Read the model definition and answer for the solid it produces. Units are mm, in the model's axes. A direction names the side the tool comes from. Coordinates: 2 decimals unless noted, no trailing zeros.
1) Find the intervals of material crossed by line 1 (X direction, y = -164.5, z = 1.3); line 2 (Y direction, x = 48, z = 2.05); line 3 (X direction, y = -137.5, z = 0.65), in increasing order.
2) Each of these flat-tipped pins is pushed along its axis until it touches: pin 1 Ø1.5 at (x, z) = (36.5, 1) entering from -Y; pin 2 Ø0.9 at (y, z) = (-146.5, 2) entering from -X; pin 3 Ø0.8 at (x, z) = (0, 1.5) entering from -Y. Where does it stop, or does it pass through?
3) Which of the six approach directions +Z, -Z, +X, -X, +Y, -Y give full straight-line access (tool end or side, diameter ignored) to faces 5 (the face through (-207.952, 49.047, 1.479)), 6 (the face through (146.452, 155.568, 1.479)), 7 (the face through (105, -170, 1))?
4) Determine the mould class of faces 1 (the face through (-148.97, 188.17, 1.48)), 2 (the face through (83.435, 73.401, 1.479)), 3 (the face through (-152, -145, 1)), 4 (the face through (-3, -10, 3)) for opening direction X: +X half, -X half, draft (parallel to the pull), parting line (faces both ways), or undercut.
Autodesk Fusion 360 part; units mm, degrees
sketch "Esboço1" plane through (0, 0, 0) normal (0, 0, 1) x (1, 0, 0)
  circle A0 centre (0, 0) radius 240
  line L0 (48, -48) -> (-48, -48)
  line L1 (-48, -48) -> (-48, 48)
  line L2 (-48, 48) -> (48, 48)
  line L3 (48, 48) -> (48, -48)
  line L4 (48, -48) -> (-48, 48) construction
  line L5 (-48, -48) -> (48, 48) construction
  circle A1 centre (-48, 48) radius 5
  circle A2 centre (-48, -48) radius 5
  circle A3 centre (48, 48) radius 5
  circle A4 centre (48, -48) radius 5
  line L6 (105, -110) -> (105, -170)
  line L7 (90, -125) -> (90, -155)
  line L8 (120, -125) -> (120, -155)
  arc A5 (120, -125) -> (90, -125) centre (105, -125) ccw
  arc A6 (90, -155) -> (120, -155) centre (105, -155) ccw
  circle A7 centre (148, -148) radius 5
  line L9 (-125, 204.878) -> (125, 204.878)
  circle A8 centre (0, 311.043) radius 164
  circle A9 centre (107.5, 130.5) radius 5
  line L10 (-40, 115) -> (40, 115)
  line L11 (-40, 115) -> (-40, 151.9958)
  line L12 (40, 115) -> (40, 151.9958)
  line L13 (0, 1.75) -> (0, 22.5)
  line L14 (-120, -125) -> (-120, -155)
  arc A10 (-90, -125) -> (-120, -125) centre (-105, -125) ccw
  line L15 (-90, -125) -> (-90, -155)
  arc A11 (-120, -155) -> (-90, -155) centre (-105, -155) ccw
  circle A12 centre (-148, -148) radius 5
  circle A13 centre (-107.5, 130.5) radius 5
  line L16 (-61.5, -178) -> (61.5, -178)
  line L17 (61.5, -178) -> (61.5, -240)
  line L18 (61.5, -240) -> (-61.5, -240)
  line L19 (-61.5, -240) -> (-61.5, -178)
  line L20 (0, -178) -> (0, -168)
  line L21 (-37.5, -168) -> (37.5, -168)
  circle A14 centre (-37.5, -168) radius 2.5
  circle A15 centre (37.5, -168) radius 2.5
  circle A16 centre (37.5, -108) radius 2.5
  circle A17 centre (37.5, -48) radius 2.5
  circle A18 centre (-37.5, -108) radius 2.5
  circle A19 centre (-37.5, -48) radius 2.5
  circle A20 centre (126.7423, 116.476) radius 2.5
  line L22 (238.5961, 66.7394) -> (184.9025, 35.7394)
  line L23 (184.9025, 35.7394) -> (123.4025, 142.2606)
  line L24 (123.4025, 142.2606) -> (177.0961, 173.2606)
  circle A21 centre (74.7807, 86.476) radius 2.5
  circle A22 centre (164.2423, 51.524) radius 2.5
  circle A23 centre (112.2807, 21.524) radius 2.5
  circle A24 centre (60.3192, -8.476) radius 2.5
  circle A25 centre (22.8192, 56.476) radius 2.5
  circle A26 centre (-164.2423, 51.524) radius 2.5
  line L25 (-177.0961, 173.2606) -> (-123.4025, 142.2606)
  line L26 (-123.4025, 142.2606) -> (-184.9025, 35.7394)
  line L27 (-184.9025, 35.7394) -> (-238.5961, 66.7394)
  circle A27 centre (-112.2807, 21.524) radius 2.5
  circle A28 centre (-126.7423, 116.476) radius 2.5
  circle A29 centre (-74.7807, 86.476) radius 2.5
  circle A30 centre (-22.8192, 56.476) radius 2.5
  circle A31 centre (-60.3192, -8.476) radius 2.5
  line L28 (0, -178) -> (0, -153)
  line L29 (-22.5, -153) -> (22.5, -153)
  circle A32 centre (-22.5, -153) radius 5
  circle A33 centre (22.5, -153) radius 5
  circle A34 centre (-22.5, -104) radius 5
  circle A35 centre (22.5, -104) radius 5
  circle A36 centre (143.7519, 57.0144) radius 5
  circle A37 centre (101.3166, 32.5144) radius 5
  circle A38 centre (78.8166, 71.4856) radius 5
  circle A39 centre (121.2519, 95.9856) radius 5
  circle A40 centre (-121.2519, 95.9856) radius 5
  circle A41 centre (-78.8166, 71.4856) radius 5
  circle A42 centre (-101.3166, 32.5144) radius 5
  circle A43 centre (-143.7519, 57.0144) radius 5
  line L30 (-17.902, -72) -> (18.098, -72)
  circle A44 centre (-17.902, -72) radius 1.75
  circle A45 centre (18.098, -72) radius 1.75
  line L31 (0, 311.043) -> (0, 115)
  circle A46 centre (-17.902, 74) radius 1.75
  circle A47 centre (18.098, 74) radius 1.75
  point P0 (105, -110)
  point P1 (0, 115)
  point P2 (0, -240)
  point P3 (-61.5, -231.9865)
  point P4 (-170.1562, 169.2538)
  point P5 (170.1562, 169.2538)
  point P6 (0.098, -72)
  dimension "d1" = 480
  dimension "d2" = 96
  dimension "d3" = 96
  dimension "d4" = 10
  dimension "d5" = 10
  dimension "d6" = 10
  dimension "d7" = 10
  dimension "d8" = 110
  dimension "d9" = 105
  dimension "d10" = 30
  dimension "d11" = 60
  dimension "d12" = 30
  dimension "d13" = 10
  dimension "d14" = 148
  dimension "d15" = 148
  dimension "d16" = 250
  dimension "d17" = 328
  dimension "d18" = 10
  dimension "d19" = 130.5
  dimension "d20" = 107.5
  dimension "d21" = 115
  dimension "d22" = 80
  dimension "d25" = 123
  dimension "d26" = 62
  dimension "d27" = 10
  dimension "d28" = 75
  dimension "d29" = 5
  dimension "d30" = 5
  dimension "d33" = 1
  dimension "d34" = 60
  dimension "d36" = 360
  dimension "d37" = 25
  dimension "d38" = 45
  dimension "d39" = 10
  dimension "d40" = 10
  dimension "d43" = 0
  dimension "d44" = 49
  dimension "d45" = 36
  dimension "d46" = 3.5
  dimension "d47" = 3.5
  dimension "d51" = 0
  dimension "d52" = 146
  dimension "d53" = 32
extrude "Extrusão1" add sketch "Esboço1" along normal blind 3 contours A0 A8 L10 L11 L12 L16 L17 L19 L22 L23 L24 L25 L26 L27 | A8 L10 L12 L31 | A8 L10 L11 L31 | L0 L1 L2 L3 A1 A2 A3 A4 A17 A19 | L0 A19 | L0 A17 picked at (-37.3146, -47.1876) picked at (37.6854, -47.1876)
sketch "Esboço2" plane through (0, -178, 0) normal (0, -1, 0) x (1, 0, 0)
  line L0 (-61.5, 0) -> (61.5, 0)
  line L1 (61.5, 0) -> (61.5, 3)
  line L2 (61.5, 3) -> (-61.5, 3)
  line L3 (-61.5, 3) -> (-61.5, 0)
  line L4 (-61.5, 3) -> (61.5, 3)
  line L5 (61.5, 3) -> (61.5, 0)
  line L6 (61.5, 0) -> (-61.5, 0)
  line L7 (-61.5, 0) -> (-61.5, 3)
  line L8 (0, 3) -> (0, 0)
  line L9 (-61.5, 1.5) -> (61.5, 1.5)
  circle A0 centre (0, 1.5) radius 0.75
  dimension "d54" = 1.5
sketch "Esboço3" plane through (154.1525, 89, 0) normal (0.866, 0.5, 0) x (-0.5, 0.866, 0)
  line L0 (-61.5, 0) -> (61.5, 0)
  line L1 (61.5, 0) -> (61.5, 3)
  line L2 (61.5, 3) -> (-61.5, 3)
  line L3 (-61.5, 3) -> (-61.5, 0)
  line L4 (-61.5, 3) -> (61.5, 3)
  line L5 (61.5, 3) -> (61.5, 0)
  line L6 (61.5, 0) -> (-61.5, 0)
  line L7 (-61.5, 0) -> (-61.5, 3)
  line L8 (-61.5, 1.5) -> (61.5, 1.5)
  line L9 (0, 3) -> (0, 0)
  circle A0 centre (0, 1.5) radius 0.75
  dimension "d55" = 1.5
sketch "Esboço4" plane through (-154.1525, 89, 0) normal (-0.866, 0.5, 0) x (-0.5, -0.866, 0)
  line L0 (-61.5, 0) -> (61.5, 0)
  line L1 (61.5, 0) -> (61.5, 3)
  line L2 (61.5, 3) -> (-61.5, 3)
  line L3 (-61.5, 3) -> (-61.5, 0)
  line L4 (-61.5, 3) -> (61.5, 3)
  line L5 (61.5, 3) -> (61.5, 0)
  line L6 (61.5, 0) -> (-61.5, 0)
  line L7 (-61.5, 0) -> (-61.5, 3)
  line L8 (0, 3) -> (0, 0)
  line L9 (-61.5, 1.5) -> (61.5, 1.5)
  circle A0 centre (0, 1.5) radius 0.75
  dimension "d56" = 1.5
extrude "Extrusão2" add sketch "Esboço4" along normal blind 5 contours L8 L9 A0 | L8 L9 A0 | L8 L9 A0 | L8 L9 A0
extrude "Extrusão3" add sketch "Esboço2" along normal blind 5 contours L8 L9 A0 | L8 L9 A0 | L8 L9 A0 | L8 L9 A0
extrude "Extrusão4" add sketch "Esboço3" along normal blind 5 contours L8 L9 A0 | L8 L9 A0 | L8 L9 A0 | L8 L9 A0
equation "d12 = d10"
equation "d17 = ( 164 * 2 ) * 1 mm"
Reported:
1. line 1: x = -174.76 to -116.61, -93.39 to 93.39, 116.61 to 174.76
1. line 2: y = -178 to -53, -43 to 43, 53 to 154.22
1. line 3: x = -196.71 to -120, -90 to 90, 120 to 196.71
2. pin 1: stops at y = -178
2. pin 2: stops at x = -190.45
2. pin 3: stops at y = -183
3. face 5: +Z, -Z, +Y
3. face 6: +Z, -Z, +X
3. face 7: +Z, -Z
4. face 1: -X half
4. face 2: undercut
4. face 3: undercut
4. face 4: draft
